```python
from build123d import *

# Parameters (mm, degrees)
SKETCH1_R           = 23.495
SKETCH1_R_2         = 2.499995
SKETCH1_R_3         = 2.54
BOSS_EXTRUDE1_DEPTH = 3.175


with BuildPart() as part:
    # Sketch1 → Boss-Extrude1 (new body)
    with BuildSketch(Plane(origin=(0, 0, 0), x_dir=(1, 0, 0), z_dir=(0, 1, 0))):
        with BuildLine():
            Line((-13.993314597, 28.4999938), (-25.9599938, 28.4999938))
            ThreePointArc((-25.9599938, 28.4999938), (-27.756045024, 27.756045024), (-28.4999938, 25.9599938))
            Line((-28.4999938, 25.9599938), (-28.4999938, 13.993314597))
            Line((-28.4999938, 13.993314597), (-28.4999938, 9.525))
            Line((-28.4999938, 9.525), (-36.1199938, 9.525))
            ThreePointArc((-36.1199938, 9.525), (-39.712096248, 8.037102448), (-41.1999938, 4.445))
            Line((-41.1999938, 4.445), (-41.1999938, -4.445))
            ThreePointArc((-41.1999938, -4.445), (-39.712096248, -8.037102448), (-36.1199938, -9.525))
            Line((-36.1199938, -9.525), (-28.4999938, -9.525))
            Line((-28.4999938, -9.525), (-28.4999938, -13.993314597))
            Line((-28.4999938, -13.993314597), (-28.4999938, -25.9599938))
            ThreePointArc((-28.4999938, -25.9599938), (-27.756045024, -27.756045024), (-25.9599938, -28.4999938))
            Line((-25.9599938, -28.4999938), (-13.993314597, -28.4999938))
            Line((-13.993314597, -28.4999938), (13.993314597, -28.4999938))
            Line((13.993314597, -28.4999938), (25.9599938, -28.4999938))
            ThreePointArc((25.9599938, -28.4999938), (27.756045024, -27.756045024), (28.4999938, -25.9599938))
            Line((28.4999938, -25.9599938), (28.4999938, -13.993314597))
            Line((28.4999938, -13.993314597), (28.4999938, -9.525))
            Line((28.4999938, -9.525), (36.1199938, -9.525))
            ThreePointArc((36.1199938, -9.525), (39.712096248, -8.037102448), (41.1999938, -4.445))
            Line((41.1999938, -4.445), (41.1999938, 4.445))
            ThreePointArc((41.1999938, 4.445), (39.712096248, 8.037102448), (36.1199938, 9.525))
            Line((36.1199938, 9.525), (28.4999938, 9.525))
            Line((28.4999938, 9.525), (28.4999938, 13.993314597))
            Line((28.4999938, 13.993314597), (28.4999938, 25.9599938))
            ThreePointArc((28.4999938, 25.9599938), (27.756045024, 27.756045024), (25.9599938, 28.4999938))
            Line((25.9599938, 28.4999938), (13.993314597, 28.4999938))
            Line((13.993314597, 28.4999938), (-13.993314597, 28.4999938))
        make_face()
        Circle(SKETCH1_R, mode=Mode.SUBTRACT)
        with Locations((-23.5000038, 23.5000038)):
            Circle(SKETCH1_R_2, mode=Mode.SUBTRACT)
        with Locations((23.5000038, 23.5000038)):
            Circle(SKETCH1_R_2, mode=Mode.SUBTRACT)
        with Locations((23.5000038, -23.5000038)):
            Circle(SKETCH1_R_2, mode=Mode.SUBTRACT)
        with Locations((-23.5000038, -23.5000038)):
            Circle(SKETCH1_R_2, mode=Mode.SUBTRACT)
        with Locations((-34.8499938, 0)):
            Circle(SKETCH1_R_3, mode=Mode.SUBTRACT)
        with Locations((34.8499938, 0)):
            Circle(SKETCH1_R_3, mode=Mode.SUBTRACT)
    extrude(amount=BOSS_EXTRUDE1_DEPTH)


solid = part.part
```
Geometry: final body of the model. Coordinates: model frame, mm. A direction names the side the tool comes from. Coordinates: 2 decimals unless noted, no trailing zeros. Write each loop counter-clockwise with the first axis right and the second up, starting at its lowest first coordinate (ties: lowest second). Pieces come first, ordered by that corner, then holes. Notation, with made-up numbers: M 14.25,-8 L 20.25,-8 A16 ccw 20.25,-3 Z; hole C 79.25,-33.75 d7. An arc over 180 degrees is marked long. Use CSV: the item, a comma, the result in double quotes. Start each with the question number.
1. Ray query, probe 1 along X at (y, z) = (1.85, 0) (3 decimals); probe 2 along Z at (x, y) = (0, 0.95) (3 decimals); probe 3 along X at (y, z) = (1.95, 25). Return the intervals inside material, ascending.
2. Cut plane D-D on z = 16.5. Return the cut outline in (x, y) (3 decimals), plus the area to 3 significant figures.
3. Cut plane B-B on y = 2.05. Return the cut outline in (x, z) (3 decimals).
4. Mould query, pull axis Z, two halves, no side actions, for faces 6 (the face through (-32, 2, 9.525)), 7 (the face through (-5.093, 1.565, 22.936)), 8 (the face through (28.5, 2, 18)). Classes: pulls with the +Z half, pulls with the -Z half, needs draft (parallel to the pull), parting line crosses it, or undercut.
5. First-contact query: P1, Ø1.6, axis at x = 34, y = 1, coming from the -Z side (3 decimals); P2, Ø1, axis at x = -29.5, y = 0.5, coming from the +Z side (3 decimals); P3, Ø1.5, axis at y = 2, z = 7.5, coming from the +X side; P4, Ø3, axis at x = 23.5, z = -23.5, coming from the -Y side. Flat tips, straight axial feed; report the tip coordinate or a pass-through.
6. Cut plane C-C on x = 0. Return the cut outline in (y, z) (3 decimals), plus the area to 3 significant figures.
7. Reachability of faces 1 (the face through (0, 2, -28.5)), 2 (the face through (32, 2, 9.525)), 3 (the face through (25.885, 1.565, 22.749)), 4 (the face through (32, 2, -9.525)), 5 (the face through (-28.5, 2, -18)) from +Z, -Z, +X, -X, +Y, -Y: full face, straight path, thin tool, end or side. Return the list, or none.
8. Cut plane A-A on z = 0. Return the cut outline in (x, y) (3 decimals).
Entries:
1,probe 1,"-41.2 to -37.39, -32.31 to -23.495, 23.495 to 32.31, 37.39 to 41.2"
1,probe 2,"-28.5 to -23.495, 23.495 to 28.5"
1,probe 3,"-28.5 to -25.5, -21.5 to 21.5, 25.5 to 28.5"
2,outline,"M -28.5,0 L -16.726,0 L -16.726,3.175 L -28.5,3.175 Z; M 16.726,0 L 28.5,0 L 28.5,3.175 L 16.726,3.175 Z"
2,area,"74.8 mm²"
3,outline,"M -41.2,-4.445 A5.08 ccw -36.12,-9.525 L -28.5,-9.525 L -28.5,-25.96 A2.54 ccw -25.96,-28.5 L 25.96,-28.5 A2.54 ccw 28.5,-25.96 L 28.5,-9.525 L 36.12,-9.525 A5.08 ccw 41.2,-4.445 L 41.2,4.445 A5.08 ccw 36.12,9.525 L 28.5,9.525 L 28.5,25.96 A2.54 ccw 25.96,28.5 L -25.96,28.5 A2.54 ccw -28.5,25.96 L -28.5,9.525 L -36.12,9.525 A5.08 ccw -41.2,4.445 Z; hole C -34.85,0 d5.08; hole C -23.5,-23.5 d5; hole C -23.5,23.5 d5; hole C 0,0 d46.99; hole C 23.5,-23.5 d5; hole C 23.5,23.5 d5; hole C 34.85,0 d5.08"
4,face 6,"pulls with the +Z half"
4,face 7,"undercut"
4,face 8,"needs draft"
5,P1,"z = -9.525"
5,P2,"z = 9.525"
5,P3,"x = 40.65"
5,P4,"through"
6,outline,"M 0,-28.5 L 3.175,-28.5 L 3.175,-23.495 L 0,-23.495 Z; M 0,23.495 L 3.175,23.495 L 3.175,28.5 L 0,28.5 Z"
6,area,"31.8 mm²"
7,face 1,"-Z, +X, -X, +Y, -Y"
7,face 2,"+Z, +X, +Y, -Y"
7,face 3,"+Y, -Y"
7,face 4,"-Z, +X, +Y, -Y"
7,face 5,"-Z, -X, +Y, -Y"
8,outline,"M -41.2,0 L -37.39,0 L -37.39,3.175 L -41.2,3.175 Z; M -32.31,0 L -23.495,0 L -23.495,3.175 L -32.31,3.175 Z; M 23.495,0 L 32.31,0 L 32.31,3.175 L 23.495,3.175 Z; M 37.39,0 L 41.2,0 L 41.2,3.175 L 37.39,3.175 Z"
